Verification items for the finished model (mm, model axes). Face numbers are marked on the shaded views. Give positions to 0.01 mm unless a question says otherwise; leave off trailing zeros. Order: outer loops, then holes, each group sorted by start corner. A loop starts at its lowest first (then second) coordinate and runs counter-clockwise, first axis right, second up.
Autodesk Inventor part; units mm, degrees
ref_plane "YZ Plane" through (0, 0, 0) normal (1, 0, 0) x (0, 1, 0)
ref_plane "XZ Plane" through (0, 0, 0) normal (0, 1, 0) x (-1, 0, 0)
ref_plane "XY Plane" through (0, 0, 0) normal (0, 0, 1) x (1, 0, 0)
sketch "Sketch1" plane through (0, 0, 0) normal (0, 0, 1) x (1, 0, 0)
  circle A0 centre (0, 0) radius 3
  line L0 (0.852, 2.8765) -> (11.2, -0.1887)
  line L1 (11.2, -0.1887) -> (11.2, -3.1887)
  line L2 (11.2, -3.1887) -> (2.9091, -0.7329)
  line L3 (0, 0) -> (-3, 0) construction
  dimension "d0" = 11.2
  dimension "d1" = 16.5
  dimension "d2" = 6
  dimension "d3" = 3
extrude "Extrusion1" add sketch "Sketch1" along normal blind 1.5
fillet "Fillet1" radius 0.5 3 edges at (2.9091, -0.7329, 0.75) (11.2, -3.1887, 0.75) (11.2, -0.1887, 0.75)
sketch "Sketch2" plane through (0, 0, 1.5) normal (0, 0, 1) x (1, 0, 0)
  line L0 (10.558, -2.9986) -> (3.3715, -0.8698)
  point P0 (0, 0)
  point P1 (6.3, -0.2772)
  dimension "d7" = 1.4
  dimension "d8" = 6.3
hole "Hole1" at (6.3, -0.2772, 1.5) direction (0, 0, -1) diameter 1.5 end through all
hole "Hole2" at (0, 0, 1.5) direction (0, 0, -1) diameter 3 end through all
fillet "Fillet2" radius 0.3 14 edges at (11.1006, -0.2629, 1.5) (11.2, -1.5406, 1.5) (10.9992, -2.9198, 1.5) (6.9647, -1.9342, 1.5) (3.0149, -0.8976, 1.5) (-2.7097, -1.2874, 1.5) (5.847, 1.3969, 1.5) (10.9992, -2.9198, 0) (11.2, -1.5406, 0) (11.1006, -0.2629, 0) (5.847, 1.3969, 0) (-2.7097, -1.2874, 0) (3.0149, -0.8976, 0) (6.9647, -1.9342, 0)
properties part number "403-05" material "Steel, Mild"
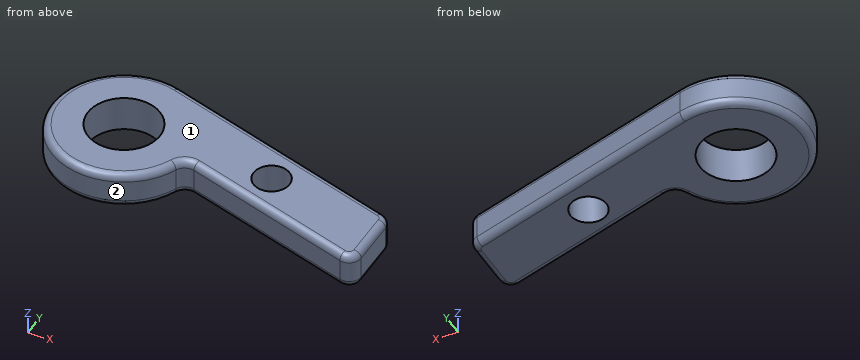
(1) Release check for a two-part mould opening along X. For the marked faces 1 and 2 record: pulls with the +X half, pulls with the -X half, needs draft (parallel to the pull), parting line crosses it, or undercut.
Solved:
face 1: needs draft
face 2: undercut
(2) Scan lines: line 1 (Y direction, x = 0, z = 1.05); line 2 (Y direction, x = 6.5, z = 0.7); line 3 (Z direction, x = -1.5, y = 2.5). Record each from-to range of solid material in increasing order.
Solved:
line 1: y = -3 to -1.5, 1.5 to 3
line 2: y = -1.8 to -1, 0.45 to 1.2
line 3: z = 0.09 to 1.41
(3) Section check A-A, the plane x = 0. Enter the section's corners in (y, z).
Solved:
outline: (-3, 0.3) arc R0.3 ccw to (-2.7, 0) - (-1.5, 0) - (-1.5, 1.5) - (-2.7, 1.5) arc R0.3 ccw to (-3, 1.2) - close; (1.5, 0) - (2.7, 0) arc R0.3 ccw to (3, 0.3) - (3, 1.2) arc R0.3 ccw to (2.7, 1.5) - (1.5, 1.5) - close
